The model under review builds one solid part; all positions refer to its coordinate system, in mm. A direction names the side the tool comes from. Round coordinates to 2 decimals unless told otherwise and drop trailing zeros. Write each loop counter-clockwise with the first axis right and the second up, starting at its lowest first coordinate (ties: lowest second). Pieces come first, ordered by that corner, then holes. Notation, with made-up numbers: (-10, -8.5) -> (40, -8.5) arc R29 ccw to (40, 20.5) -> close; hole circle Ø2 at (75.25, -36). An arc over 180 degrees is marked (long way). Use CSV: the item, a comma, the result in double quotes. Start each with the question number.
1) Machinability: for faces 4 (the face through (-41, 55.6, 22)), 5 (the face through (-36, 31, -13)), 6 (the face through (16, 17, 5)), 7 (the face through (48, 12, 4)), 8 (the face through (17, 38, 0)), which of the approach directions +Z, -Z, +X, -X, +Y, -Y give a long, thin tool a straight path to every point of the face, cutting with its end or side? Answer none if there is none.
2) Take a section at D-D, the plane z = 18.5. Give the boundary of the cut face in (x, y), then the cut area to 3 significant figures.
3) Take a section at C-C, the plane z = 40.5. Give the boundary of the cut face in (x, y), then the cut area to 3 significant figures.
4) For pin 1 Ø4.5 at (y, z) = (1.5, -5) entering from +X; pin 2 Ø12 at (x, z) = (21.5, -5) entering from +Y; pin 3 Ø1 at (x, z) = (25, -9.5) entering from +Y; pin 4 Ø4 at (x, z) = (-57, 0) entering from +Y, all flat-tipped, find the tip position at first contact; note any pin that passes through.
5) Take a section at B-B, the plane x = -40. Give the boundary of the cut face in (y, z).
6) Wall thickness on probe 1 along X at (y, z) = (7, -0.5); probe 2 along X at (y, z) = (32, 5); probe 3 along Y at (x, z) = (47, 0): over which ranges is each line inside the solid? List them lowest first. Write a range as [from, to].
7) Take a section at A-A, the plane y = 7.5. Give the boundary of the cut face in (x, z), then the cut area to 3 significant figures.
8) Mouldability with a two-part tool opening along Z and no side actions: class faces 1 (the face through (15.02, 29.95, 47.69)), 2 (the face through (15, 0, 1)), 3 (the face through (16, 21, 13)) as released by +Z, released by -Z, zero draft, split by the parting line, or undercut.
from build123d import *

# Parameters (mm, degrees)
SKETCH1_R               = 65
SKETCH1_R_2             = 46
SKETCH1_R_3             = 1.7
BOSS_EXTRUDE1_DEPTH     = 5
SKETCH3_R               = 50
SKETCH3_R_2             = 46
BOSS_EXTRUDE2_DEPTH     = 50.6
BOSS_EXTRUDE3_DEPTH     = 4
BOSS_EXTRUDE4_DEPTH     = 8
BOSS_EXTRUDE5_DEPTH     = 38
CUT_EXTRUDE3_REACH      = 145.323
CUT_EXTRUDE3_END_RADIUS = 46
SKETCH12_R              = 5
SKETCH13_W              = 42
SKETCH13_H              = 26
CUT_EXTRUDE4_DEPTH      = 38
SKETCH14_R              = 1.3
CUT_EXTRUDE5_DEPTH      = 7.5
CUT_EXTRUDE6_DEPTH      = 25
FILLET1_R               = 1


with BuildPart() as part:
    # Sketch1 → Boss-Extrude1 (new body)
    with BuildSketch(Plane(origin=(0, 0, 0), x_dir=(1, 0, 0), z_dir=(0, 1, 0))):
        with Locations(Location((0, 0, 0), (0, 0, 270))):
            Circle(SKETCH1_R)
        with Locations(Location((0, 0, 0), (0, 0, 270))):
            Circle(SKETCH1_R_2, mode=Mode.SUBTRACT)
        with Locations(Location((0, -57, 0), (0, 0, 270))):
            Circle(SKETCH1_R_3, mode=Mode.SUBTRACT)
        with Locations(Location((-57, 0, 0), (0, 0, 270))):
            Circle(SKETCH1_R_3, mode=Mode.SUBTRACT)
        with Locations(Location((0, 57, 0), (0, 0, 270))):
            Circle(SKETCH1_R_3, mode=Mode.SUBTRACT)
        with Locations(Location((57, 0, 0), (0, 0, 270))):
            Circle(SKETCH1_R_3, mode=Mode.SUBTRACT)
    extrude(amount=BOSS_EXTRUDE1_DEPTH)

    # Sketch3 → Boss-Extrude2 (add)
    with BuildSketch(Plane(origin=(0, 5, 0), x_dir=(1, 0, 0), z_dir=(0, 1, 0))):
        with Locations(Location((0, 0, 0), (0, 0, 270))):
            Circle(SKETCH3_R)
        with Locations(Location((0, 0, 0), (0, 0, 270))):
            Circle(SKETCH3_R_2, mode=Mode.SUBTRACT)
    extrude(amount=BOSS_EXTRUDE2_DEPTH)

    # Sketch4 → Boss-Extrude3 (add)
    with BuildSketch(Plane.XZ):
        with BuildLine():
            Line((30.98386677, -34), (12.463607592, -13))
            Line((12.463607592, -13), (12.463607592, 13))
            Line((12.463607592, 13), (30.98386677, 34))
            ThreePointArc((30.98386677, 34), (46, 0), (30.98386677, -34))
        make_face()
        with BuildLine():
            Line((24.463607592, 16), (30.98386677, 23.393278972))
            ThreePointArc((30.98386677, 23.393278972), (38.823259794, 0), (30.98386677, -23.393278972))
            Line((30.98386677, -23.393278972), (24.463607592, -16))
            Line((24.463607592, -16), (24.463607592, 16))
        make_face(mode=Mode.SUBTRACT)
    extrude(amount=-BOSS_EXTRUDE3_DEPTH)

    # Sketch6 → Boss-Extrude4 (add)
    with BuildSketch(Plane.ZY.offset(-12.463607592)):
        Polygon((13, 4), (13, 38), (-13, 38), (-13, 4), (-5, 4), (-5, 28), (5, 28), (5, 4), align=None)
    extrude(amount=-BOSS_EXTRUDE4_DEPTH)

    # Sketch7 → Boss-Extrude5 (add)
    with BuildSketch(Plane.XZ):
        with BuildLine():
            Line((-44.124822946, 13), (12.463607592, 13))
            Line((12.463607592, 13), (12.463607592, -13))
            Line((12.463607592, -13), (-44.124822946, -13))
            ThreePointArc((-44.124822946, -13), (-46, 0), (-44.124822946, 13))
        make_face()
    extrude(amount=-BOSS_EXTRUDE5_DEPTH)

    # Cut-Extrude3: up to this cylinder (the profile starts outside it)
    cut_extrude3_end = Plane(origin=(0, 15, 0), z_dir=(0, -1, 0)) * Cylinder(CUT_EXTRUDE3_END_RADIUS, 383.646, mode=Mode.PRIVATE)
    # Sketch12 → Cut-Extrude3 (cut, up to the surface)
    with BuildSketch(Plane(origin=(50, 0, 0), x_dir=(0, 0, -1), z_dir=(1, 0, 0)), mode=Mode.PRIVATE) as cut_extrude3_sk1:
        with Locations((0, 15)):
            Circle(SKETCH12_R)
    cut_extrude3_tool1 = extrude(cut_extrude3_sk1.sketch, amount=-CUT_EXTRUDE3_REACH, mode=Mode.PRIVATE) - cut_extrude3_end
    add(cut_extrude3_tool1.solids().sort_by_distance((50, 15, 0))[0], mode=Mode.SUBTRACT)

    # Sketch13 → Cut-Extrude4 (cut)
    with BuildSketch(Plane(origin=(0, 38, 0), x_dir=(1, 0, 0), z_dir=(0, 1, 0))):
        with Locations((-8.536392408, 0)):
            Rectangle(SKETCH13_W, SKETCH13_H)
    extrude(amount=-CUT_EXTRUDE4_DEPTH, mode=Mode.SUBTRACT)

    # Sketch14 → Cut-Extrude5 (cut)
    with BuildSketch(Plane(origin=(0, 38, 0), x_dir=(1, 0, 0), z_dir=(0, 1, 0))):
        with Locations(Location((15.663607592, 5, 0), (0, 0, 270))):
            Circle(SKETCH14_R)
        with Locations(Location((15.663607592, -5, 0), (0, 0, 270))):
            Circle(SKETCH14_R)
        with Locations(Location((-32.736392408, 5, 0), (0, 0, 270))):
            Circle(SKETCH14_R)
        with Locations(Location((-32.736392408, -5, 0), (0, 0, 270))):
            Circle(SKETCH14_R)
    extrude(amount=-CUT_EXTRUDE5_DEPTH, mode=Mode.SUBTRACT)

    # Sketch15 → Cut-Extrude6 (cut)
    with BuildSketch(Plane.XZ):
        with BuildLine():
            Line((-44.124822946, 13), (-29.536392408, 13))
            Line((-29.536392408, 13), (-29.536392408, -13))
            Line((-29.536392408, -13), (-44.124822946, -13))
            ThreePointArc((-44.124822946, -13), (-46, 0), (-44.124822946, 13))
        make_face()
    extrude(amount=-CUT_EXTRUDE6_DEPTH, mode=Mode.SUBTRACT)

    # Fillet1
    fillet1_edges = [part.edges().sort_by_distance(p)[0] for p in [
        (-46, 25, 0),
        (20.463607592, 4, -9),
        (16.463607592, 4, -5),
        (16.463607592, 4, -13),
        (20.463607592, 4, 9),
        (16.463607592, 4, 13),
        (16.463607592, 4, 5),
        (-44.124822946, 31.5, 13),
        (-44.124822946, 31.5, -13),
    ]]
    fillet(fillet1_edges, radius=FILLET1_R)


solid = part.part
Values found:
1,face 4,"+Z, -Z, +X, -X, +Y"
1,face 5,"+Y, -Y"
1,face 6,"none"
1,face 7,"+X"
1,face 8,"+Y"
2,outline,"(-62.31, 0) -> (-42.12, 0) -> (-42.12, 55.6) -> (-46.45, 55.6) -> (-46.45, 5) -> (-62.31, 5) -> close; (17.31, 0) -> (26.67, 0) -> (26.67, 4) -> (17.31, 4) -> close; (34.13, 0) -> (62.31, 0) -> (62.31, 5) -> (46.45, 5) -> (46.45, 55.6) -> (42.12, 55.6) -> (42.12, 4) -> (34.13, 4) -> close"
2,area,"710 mm²"
3,outline,"(-50.84, 0) -> (-21.81, 0) -> (-21.81, 55.6) -> (-29.32, 55.6) -> (-29.32, 5) -> (-50.84, 5) -> close; (21.81, 0) -> (50.84, 0) -> (50.84, 5) -> (29.32, 5) -> (29.32, 55.6) -> (21.81, 55.6) -> close"
3,area,"1,050 mm²"
4,pin 1,"x = 64.94"
4,pin 2,"y = 38"
4,pin 3,"through"
4,pin 4,"y = 5"
5,outline,"(0, -51.23) -> (5, -51.23) -> (5, -30) -> (55.6, -30) -> (55.6, -22.72) -> (0, -22.72) -> close; (0, 22.72) -> (55.6, 22.72) -> (55.6, 30) -> (5, 30) -> (5, 51.23) -> (0, 51.23) -> close; (25, -13) -> (38, -13) -> (38, 13) -> (25, 13) -> close"
6,probe 1,"[-50, -46], [46, 50]"
6,probe 2,"[-49.75, -34.04], [-31.44, -29.54], [12.46, 14.36], [16.96, 20.46], [45.73, 49.75]"
6,probe 3,"[0, 10], [20, 55.6]"
7,outline,"circle Ø100 at (0, 0); (12.46, -13) -> (20.46, -13) -> (20.46, -5) -> (12.46, -5) -> close; (12.46, 5) -> (20.46, 5) -> (20.46, 13) -> (12.46, 13) -> close; hole circle Ø92 at (0, 0)"
7,area,"1,330 mm²"
8,face 1,"split by the parting line"
8,face 2,"zero draft"
8,face 3,"undercut"
